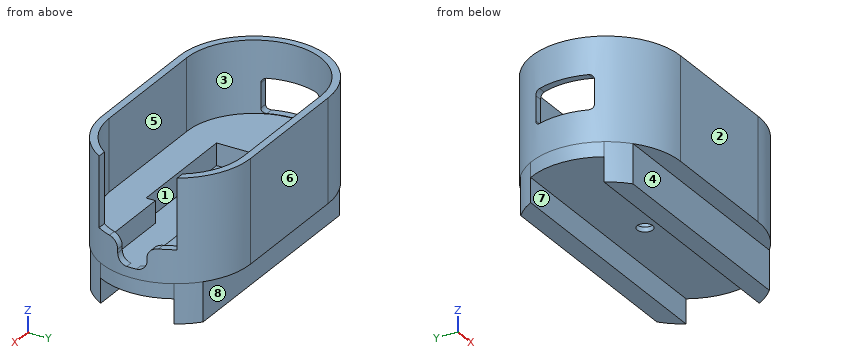
```python
from build123d import *

# Parameters (mm, degrees)
BOSS_EXTRUDE1_DEPTH = 19
BOSS_EXTRUDE2_DEPTH = 2
BOSS_EXTRUDE3_DEPTH = 4.5
SKETCH4_W           = 4.75
SKETCH4_H           = 6
SKETCH4_W_2         = 14.25
SKETCH4_H_2         = 16
CUT_EXTRUDE1_DEPTH  = 49.452157546
SKETCH5_W           = 7
SKETCH5_H           = 12
CUT_EXTRUDE2_DEPTH  = 49.452157546
FILLET1_R           = 1
SKETCH6_R           = 1.6
BOSS_EXTRUDE4_DEPTH = 3
BOSS_EXTRUDE7_DEPTH = 8
FILLET2_R           = 2
CUT_EXTRUDE3_START  = -10
SKETCH9_R           = 1.6
CUT_EXTRUDE3_DEPTH  = 10
CUT_EXTRUDE4_START  = -1
SKETCH11_R          = 2.065
CUT_EXTRUDE4_DEPTH  = 3


with BuildPart() as part:
    # Sketch1 → Boss-Extrude1 (new body)
    with BuildSketch(Plane.XY):
        with BuildLine():
            Line((-34.384444189, 18.719216619), (-7.984444189, 18.719216619))
            ThreePointArc((-7.984444189, 18.719216619), (7.265555811, 3.469216619), (-7.984444189, -11.780783381))
            Line((-7.984444189, -11.780783381), (-34.384444189, -11.780783381))
            ThreePointArc((-34.384444189, -11.780783381), (-49.634444189, 3.469216619), (-34.384444189, 18.719216619))
        make_face()
        with BuildLine():
            Line((-34.384444189, 17.219216619), (-7.984444189, 17.219216619))
            ThreePointArc((-7.984444189, 17.219216619), (5.765555811, 3.469216619), (-7.984444189, -10.280783381))
            Line((-7.984444189, -10.280783381), (-34.384444189, -10.280783381))
            ThreePointArc((-34.384444189, -10.280783381), (-48.134444189, 3.469216619), (-34.384444189, 17.219216619))
        make_face(mode=Mode.SUBTRACT)
    extrude(amount=BOSS_EXTRUDE1_DEPTH)



with BuildPart() as body_2:
    # Sketch2 → Boss-Extrude2 (new body)
    with BuildSketch(Plane(origin=(0, 0, 0), x_dir=(-1, 0, 0), z_dir=(0, 0, -1))):
        with BuildLine():
            Line((34.384444189, -11.780783381), (7.984444189, -11.780783381))
            ThreePointArc((7.984444189, -11.780783381), (-7.265555811, 3.469216619), (7.984444189, 18.719216619))
            Line((7.984444189, 18.719216619), (34.384444189, 18.719216619))
            ThreePointArc((34.384444189, 18.719216619), (49.634444189, 3.469216619), (34.384444189, -11.780783381))
        make_face()
    extrude(amount=BOSS_EXTRUDE2_DEPTH)


with BuildPart() as part_1:
    add(part.part)

    add(body_2.part)  # Boss-Extrude3 merges body 2
    # Sketch3 → Boss-Extrude3 (add)
    with BuildSketch(Plane.XY):
        with BuildLine():
            Line((-22.664695889, -3.430783381), (-33.184444189, -3.430783381))
            Line((-33.184444189, -3.430783381), (-33.184444189, 10.369216619))
            Line((-33.184444189, 10.369216619), (-19.704192488, 10.369216619))
            Line((-19.704192488, 10.369216619), (-9.184444189, 10.369216619))
            Line((-9.184444189, 10.369216619), (-9.184444189, 8.469216619))
            Line((-9.184444189, 8.469216619), (4.663184056, 8.469216619))
            ThreePointArc((4.663184056, 8.469216619), (-0.337155761, 14.715615149), (-7.984444189, 17.069308538))
            Line((-7.984444189, 17.069308538), (-34.384444189, 17.069308538))
            ThreePointArc((-34.384444189, 17.069308538), (-47.984536108, 3.469216619), (-34.384444189, -10.1308753))
            Line((-34.384444189, -10.1308753), (-7.984444189, -10.1308753))
            ThreePointArc((-7.984444189, -10.1308753), (-0.337155761, -7.777181911), (4.663184056, -1.530783381))
            Line((4.663184056, -1.530783381), (-9.184444189, -1.530783381))
            Line((-9.184444189, -1.530783381), (-9.184444189, -3.430783381))
            Line((-9.184444189, -3.430783381), (-19.704192488, -3.430783381))
            Line((-19.704192488, -3.430783381), (-22.664695889, -3.430783381))
        make_face()
    extrude(amount=BOSS_EXTRUDE3_DEPTH)

    # Sketch4 → Cut-Extrude1 (cut, through all)
    with BuildSketch(Plane.ZY.offset(9.184444189)):
        with Locations((2.375, 3.469216619)):
            Rectangle(SKETCH4_W, SKETCH4_H)
        with Locations((11.875, 3.469216619)):
            Rectangle(SKETCH4_W_2, SKETCH4_H_2)
    extrude(amount=-CUT_EXTRUDE1_DEPTH, mode=Mode.SUBTRACT)

    # Sketch5 → Cut-Extrude2 (cut, through all)
    with BuildSketch(Plane(origin=(-33.184444189, 0, 0), x_dir=(0, 0, -1), z_dir=(1, 0, 0))):
        with Locations((-8, 3.469216619)):
            Rectangle(SKETCH5_W, SKETCH5_H)
    extrude(amount=-CUT_EXTRUDE2_DEPTH, mode=Mode.SUBTRACT)

    # Fillet1
    fillet1_edges = [part_1.edges().sort_by_distance(p)[0] for p in [
        (-47.580403151, -2.530783381, 11.5),
        (-47.580403151, 9.469216619, 11.5),
        (-47.580403151, 9.469216619, 4.5),
        (-47.580403151, -2.530783381, 4.5),
    ]]
    fillet(fillet1_edges, radius=FILLET1_R)

    # Sketch6 → Boss-Extrude4 (add)
    with BuildSketch(Plane(origin=(0, 0, -2), x_dir=(-1, 0, 0), z_dir=(0, 0, -1))):
        with BuildLine():
            ThreePointArc((47.662715914, -4.030783381), (49.634444189, 3.469216619), (47.662715914, 10.969216619))
            Line((47.662715914, 10.969216619), (-5.293827536, 10.969216619))
            ThreePointArc((-5.293827536, 10.969216619), (-7.265555811, 3.469216619), (-5.293827536, -4.030783381))
            Line((-5.293827536, -4.030783381), (47.662715914, -4.030783381))
        make_face()
        with Locations((21.184444189, 3.469216619)):
            Circle(SKETCH6_R, mode=Mode.SUBTRACT)
    extrude(amount=BOSS_EXTRUDE4_DEPTH)

    # Sketch10 → Boss-Extrude7 (add)
    with BuildSketch(Plane(origin=(0, 0, -2), x_dir=(-1, 0, 0), z_dir=(0, 0, -1))):
        with BuildLine():
            Line((-5.293827536, -4.030783381), (47.662715914, -4.030783381))
            ThreePointArc((47.662715914, -4.030783381), (46.201857789, -6.169830834), (44.400057001, -8.030783381))
            Line((44.400057001, -8.030783381), (-2.031168623, -8.030783381))
            ThreePointArc((-2.031168623, -8.030783381), (-3.832969412, -6.169830834), (-5.293827536, -4.030783381))
        make_face()
        with BuildLine():
            Line((-5.293827536, 10.969216619), (47.662715914, 10.969216619))
            ThreePointArc((47.662715914, 10.969216619), (46.201857789, 13.108264072), (44.400057001, 14.969216619))
            Line((44.400057001, 14.969216619), (-2.031168623, 14.969216619))
            ThreePointArc((-2.031168623, 14.969216619), (-3.832969412, 13.108264072), (-5.293827536, 10.969216619))
        make_face()
    extrude(amount=BOSS_EXTRUDE7_DEPTH)

    # Fillet2
    fillet2_edges = [part_1.edges().sort_by_distance(p)[0] for p in [
        (6.200927538, 0.469216619, 0),
        (6.200927538, 6.469216619, 0),
        (6.200927538, 6.469216619, 4.75),
        (6.200927538, 0.469216619, 4.75),
    ]]
    fillet(fillet2_edges, radius=FILLET2_R)

    # Sketch9 → Cut-Extrude3 (cut)
    with BuildSketch(Plane(origin=(0, 0, -2), x_dir=(-1, 0, 0), z_dir=(0, 0, -1)).offset(CUT_EXTRUDE3_START)):
        with Locations((21.184444189, 3.469216619)):
            Circle(SKETCH9_R)
    extrude(amount=CUT_EXTRUDE3_DEPTH, mode=Mode.SUBTRACT)

    # Sketch11 → Cut-Extrude4 (cut)
    with BuildSketch(Plane.XY.offset(CUT_EXTRUDE4_START)):
        with Locations((-21.184444189, 3.469216619)):
            Circle(SKETCH11_R)
    extrude(amount=-CUT_EXTRUDE4_DEPTH, mode=Mode.SUBTRACT)


solid = part_1.part
```
CAD build for the part. Positions are in the model's coordinates, mm. Face numbers are marked on the shaded views. A direction names the side the tool comes from. Coordinates: 2 decimals unless noted, no trailing zeros. Loops run counter-clockwise (first coordinate to the right, second up) from the corner with the lowest first, then second, coordinate; pieces in that order, holes last. Notation, with made-up numbers: (38.5, 86) - (59.5, 86) arc R24 ccw to (59.5, 112) - close; hole circle Ø9 at (-20, 74.5). An arc over 180 degrees is marked (long way). Return JSON: item names as keys, results as strings.
1. 3-axis set-ups, long thin cutter, end or side, ignore diameter. For the marked faces 4, 5, 6, 7 and 8: which of +Z, -Z, +X, -X, +Y, -Y reach the whole face in a straight line?
Result:
{"face 4": "-Z, +X, -X, -Y", "face 5": "+Z", "face 6": "+Z, -Z, +X, -X, +Y", "face 7": "-Z, +X, -X", "face 8": "-Z, +X, -X, +Y"}
2. Probe L1, parallel to Y at x = -45, z = 2.75; L2, parallel to Y at x = -33.5, z = -8.25; L3, parallel to Y at x = -20, z = 17.25. List the from-to ranges inside material, lowest first. Write a range as from..to.
Result:
{"L1": "y = -7.48..-5.27, -5.03..11.97, 12.21..14.42", "L2": "y = -8.03..-4.03, 10.97..14.97", "L3": "y = -11.78..-10.28, 17.22..18.72"}
3. Mould opens along X. For the marked faces 1, 2 and 3 say: released by +X, released by -X, zero draft, split by the parting line, or undercut.
Result:
{"face 1": "undercut", "face 2": "zero draft", "face 3": "undercut"}
4. Band-saw the part on D-D (x = -39.5). Give the cut face in (y, z).
Result:
{"outline": "(-10.9, -2) - (-8.03, -2) - (-8.03, -10) - (-4.03, -10) - (-4.03, -5) - (10.97, -5) - (10.97, -10) - (14.97, -10) - (14.97, -2) - (17.84, -2) - (17.84, 19) - (16.23, 19) - (16.23, 0) - (16.07, 0) - (16.07, 4.5) - (-9.13, 4.5) - (-9.13, 0) - (-9.29, 0) - (-9.29, 19) - (-10.9, 19) - close"}
5. Band-saw the part on A-A (x = -12). Give the cut face in (y, z), and give its area (3 significant figures).
Result:
{"outline": "(-11.78, -2) - (-8.03, -2) - (-8.03, -10) - (-4.03, -10) - (-4.03, -5) - (10.97, -5) - (10.97, -10) - (14.97, -10) - (14.97, -2) - (18.72, -2) - (18.72, 19) - (17.22, 19) - (17.22, 0) - (17.07, 0) - (17.07, 4.5) - (10.37, 4.5) - (10.37, 0) - (-3.43, 0) - (-3.43, 4.5) - (-10.13, 4.5) - (-10.13, 0) - (-10.28, 0) - (-10.28, 19) - (-11.78, 19) - close", "area": "287 mm2"}
6. Drop flat-ended pins along their axis: pin 1 (1.5 mm diameter, centred on y = -7, z = 6.5, fed in from +X); pin 2 (9 mm diameter, centred on x = -31.5, z = -7.5, fed in from +Y); pin 3 (6 mm diameter, centred on y = -3.5, z = 1, fed in from +X); pin 4 (8 mm diameter, centred on y = 5, z = -1.5, fed in from -X). Give the stop position or say it passes through.
Result:
{"pin 1": "stops at x = 3.77", "pin 2": "stops at y = 14.97", "pin 3": "stops at x = 6.74", "pin 4": "stops at x = -49.63"}
7. Band-saw the part on C-C (y = 13.5). Give the cut face in (x, z), and give its area (3 significant figures).
Result:
{"outline": "(-45.87, -10) - (3.5, -10) - (3.5, 19) - (1.42, 19) - (1.42, 0) - (1.2, 0) - (1.2, 4.5) - (-43.57, 4.5) - (-43.57, 0) - (-43.79, 0) - (-43.79, 19) - (-45.87, 19) - close", "area": "774 mm2"}
8. Band-saw the part on B-B (z = 13.75). Give the cut face in (x, y), and give its area (3 significant figures).
Result:
{"outline": "(-34.38, -11.78) - (-7.98, -11.78) arc R15.25 ccw to (5, -4.53) - (3.2, -4.53) arc R13.75 cw to (-7.98, -10.28) - (-34.38, -10.28) arc R13.75 cw to (-34.38, 17.22) - (-7.98, 17.22) arc R13.75 cw to (3.2, 11.47) - (5, 11.47) arc R15.25 ccw to (-7.98, 18.72) - (-34.38, 18.72) arc R15.25 ccw to start", "area": "190 mm2"}
